Work out the finished part from the listing and answer in its coordinate system (mm). A direction names the side the tool comes from. Coordinates: 2 decimals unless noted, no trailing zeros. Order: outer loops, then holes, each group sorted by start corner. A loop starts at its lowest first (then second) coordinate and runs counter-clockwise, first axis right, second up. Notation, with made-up numbers: (37.25, 82) -> (69.25, 82) arc R20 cw to (69.25, 101) -> close; hole circle Ø9 at (9, 56.25). An arc over 180 degrees is marked (long way). Use one line per item in the form item = value.
from build123d import *

# Parameters (mm, degrees)
ESQUISSE1_W             = 72
ESQUISSE1_H             = 8
BOSS_EXTRU_1_DEPTH      = 50
ESQUISSE2_R             = 15
ESQUISSE2_R_2           = 13
ENL_V_MAT_EXTRU_1_DEPTH = 5
ESQUISSE3_R             = 1.5
ENL_V_MAT_EXTRU_2_DEPTH = 10
ESQUISSE4_R             = 1.5
ENL_V_MAT_EXTRU_3_DEPTH = 10
ESQUISSE5_R             = 1.5
ENL_V_MAT_EXTRU_4_DEPTH = 51


with BuildPart() as part:
    # Esquisse1 → Boss.-Extru.1 (new body)
    with BuildSketch(Plane.XY):
        with Locations((30.5, -49)):
            Rectangle(ESQUISSE1_W, ESQUISSE1_H)
    extrude(amount=BOSS_EXTRU_1_DEPTH)

    # Esquisse2 → Enlèv. mat.-Extru.1 (cut)
    with BuildSketch(Plane(origin=(0, -45, 0), x_dir=(-1, 0, 0), z_dir=(0, 1, 0))):
        with Locations((-30.5, 25)):
            Circle(ESQUISSE2_R)
        with Locations((-30.5, 25)):
            Circle(ESQUISSE2_R_2, mode=Mode.SUBTRACT)
    extrude(amount=-ENL_V_MAT_EXTRU_1_DEPTH, mode=Mode.SUBTRACT)

    # Esquisse3 → Enlèv. mat.-Extru.2 (cut)
    with BuildSketch(Plane.ZY.offset(5.5)):
        with Locations((12.5, -47.5)):
            Circle(ESQUISSE3_R)
        with Locations((37.5, -47.5)):
            Circle(ESQUISSE3_R)
    extrude(amount=-ENL_V_MAT_EXTRU_2_DEPTH, mode=Mode.SUBTRACT)

    # Esquisse4 → Enlèv. mat.-Extru.3 (cut)
    with BuildSketch(Plane(origin=(66.5, 0, 0), x_dir=(0, 0, -1), z_dir=(1, 0, 0))):
        with Locations((-37.5, -47.5)):
            Circle(ESQUISSE4_R)
        with Locations((-12.5, -47.5)):
            Circle(ESQUISSE4_R)
    extrude(amount=-ENL_V_MAT_EXTRU_3_DEPTH, mode=Mode.SUBTRACT)

    # Esquisse5 → Enlèv. mat.-Extru.4 (cut, through all)
    with BuildSketch(Plane(origin=(0, 0, 0), x_dir=(-1, 0, 0), z_dir=(0, 0, -1))):
        with Locations((-30.5, -47.5)):
            Circle(ESQUISSE5_R)
    extrude(amount=-ENL_V_MAT_EXTRU_4_DEPTH, mode=Mode.SUBTRACT)


solid = part.part
(1) Section C-C on y = -47.5 is taken. Count the separate pieces of the cut face and the enclosed holes in it, plus the area to 3 significant figures.
Data:
separate_pieces = 4
enclosed_holes = 0
area = 3,170 mm²
(2) Section B-B on x = 1.5 is taken. Write down the section's boundary in (y, z), plus the area to 3 significant figures.
Data:
outline = (-53, 0) -> (-45, 0) -> (-45, 50) -> (-53, 50) -> close; hole circle Ø3 at (-47.5, 12.5); hole circle Ø3 at (-47.5, 37.5)
area = 386 mm²
(3) Section A-A on z = 25 is taken. Write down the section's boundary in (x, y), plus the area to 3 significant figures.
Data:
outline = (-5.5, -53) -> (66.5, -53) -> (66.5, -45) -> (45.5, -45) -> (45.5, -50) -> (43.5, -50) -> (43.5, -45) -> (17.5, -45) -> (17.5, -50) -> (15.5, -50) -> (15.5, -45) -> (-5.5, -45) -> close; hole circle Ø3 at (30.5, -47.5)
area = 549 mm²
(4) Section D-D on x = 24 is taken. Write down the section's boundary in (y, z).
Data:
outline = (-53, 0) -> (-45, 0) -> (-45, 11.48) -> (-50, 11.48) -> (-50, 13.74) -> (-45, 13.74) -> (-45, 36.26) -> (-50, 36.26) -> (-50, 38.52) -> (-45, 38.52) -> (-45, 50) -> (-53, 50) -> close
(5) Each of these flat-tipped pins is pushed along its axis until it touches: P1, Ø3, axis at x = 52.5, y = -48.5, coming from the -Z side; P2, Ø0.9, axis at y = -47.5, z = 37, coming from the +X side; P3, Ø1.5, axis at y = -48, z = 37.5, coming from the -X side. Where does it stop, or does it pass through?
Data:
P1 = 0
P2 = 56.5
P3 = 4.5
(6) Which of the six approach directions +Z, -Z, +X, -X, +Y, -Y give full straight-line access (tool end or side, diameter ignored) to faces 5 (the cylindrical face through (43.487, -47.465, 25.572)), 6 (the cylindrical face through (61.57, -48.964, 37.825)), 7 (the flat face through (4.5, -47, 37))?
Data:
face_5 = +Y
face_6 = +X
face_7 = -X
(7) The mould has two halves that part along X. Classify faces 1 (the flat face through (66.5, -49, 25)), 2 (the flat face through (42, -50, 32)), 3 (the cylindrical face through (-0.57, -48.964, 37.175)), 4 (the cylindrical face through (30.825, -48.964, 24.818)): released by +X, released by -X, zero draft, split by the parting line, or undercut.
Data:
face_1 = released by +X
face_2 = undercut
face_3 = zero draft
face_4 = undercut
(8) Straight lines are drawn through the part: line 1 along Y through (x, z) = (30.5, 30.25); line 2 along Z through (x, y) = (22, -46.25); line 3 along Z through (x, y) = (41.5, -49). For each, find the intervals that lie inside material, in ascending order.
Data:
line_1 = -53 to -49, -46 to -45
line_2 = 0 to 12.64, 15.16 to 34.84, 37.36 to 50
line_3 = 0 to 14.8, 18.07 to 31.93, 35.2 to 50
